```python
from build123d import *

# Parameters (mm, degrees)
ESQUISSE1_R        = 2.5
ESQUISSE1_R_2      = 1.5
BOSS_EXTRU_1_DEPTH = 3.15


with BuildPart() as part:
    # Esquisse1 → Boss.-Extru.1 (new body)
    with BuildSketch(Plane.XY):
        Polygon((3.25, 0), (5.225, -7), (16.275, -7), (18.25, 0), (21.5, 0), (21.5, 22.15), (0, 22.15), (0, 0), align=None)
        with Locations((10.75, 11.075)):
            Circle(ESQUISSE1_R, mode=Mode.SUBTRACT)
        with Locations((10.75, -1.5)):
            Circle(ESQUISSE1_R_2, mode=Mode.SUBTRACT)
    extrude(amount=BOSS_EXTRU_1_DEPTH)


solid = part.part
```
Input: part model. Units: mm. Frame: model coordinates. A direction names the side the tool comes from. Give positions to 0.01 mm unless a question says otherwise; leave off trailing zeros. Order: outer loops, then holes, each group sorted by start corner. A loop starts at its lowest first (then second) coordinate and runs counter-clockwise, first axis right, second up. Notation, with made-up numbers: (25, 44) - (69, 44) arc R24 cw to (69, 66) - close; hole circle Ø5 at (62, -32.5). An arc over 180 degrees is marked (long way). Put each result on its own line as item: value.
Item 1: Draft query along Y for faces 1 (the cylindrical face through (8.907, 12.765, 1.553)), 2 (the flat face through (11, 8, 3.15)), 3 (the flat face through (20, 0, 2)). Return one class per face: +Y half, -Y half, draft (parallel to the pull), parting line (faces both ways), or undercut.
Found:
face 1: undercut
face 2: draft
face 3: -Y half
Item 2: Section query A-A, the plane y = 10.5. Return loops of the section in (x, z).
Found:
outline: (0, 0) - (8.32, 0) - (8.32, 3.15) - (0, 3.15) - close; (13.18, 0) - (21.5, 0) - (21.5, 3.15) - (13.18, 3.15) - close
Item 3: Ray query, L1, parallel to Y at x = 10.75, z = 0.7 (3 decimals); L2, parallel to Y at x = 11.75, z = 2.75; L3, parallel to X at y = 11.75, z = 1.55. Return the intervals inside material, ascending. Write a range as from..to.
Found:
L1: y = -7..-3, 0..8.575, 13.575..22.15
L2: y = -7..-2.62, -0.38..8.78, 13.37..22.15
L3: x = 0..8.34, 13.16..21.5
Item 4: Section query B-B, the plane x = 10.75. Return loops of the section in (y, z) (3 decimals).
Found:
outline: (-7, 0) - (-3, 0) - (-3, 3.15) - (-7, 3.15) - close; (0, 0) - (8.575, 0) - (8.575, 3.15) - (0, 3.15) - close; (13.575, 0) - (22.15, 0) - (22.15, 3.15) - (13.575, 3.15) - close
Item 5: Access query for faces 4 (the flat face through (2, 0, 2)), 5 (the cylindrical face through (9.25, -1.43, 1.55)). Directions: +Z, -Z, +X, -X, +Y, -Y. A direction counts if a zero-diameter tool reaches every point of the face in a straight line with its end or side. Return the directions, or none.
Found:
face 4: +Z, -Z, -X, -Y
face 5: +Z, -Z
Item 6: Section query D-D, the plane y = -1.5. Return loops of the section in (x, z), then the cut area to 3 significant figures.
Found:
outline: (3.67, 0) - (9.25, 0) - (9.25, 3.15) - (3.67, 3.15) - close; (12.25, 0) - (17.83, 0) - (17.83, 3.15) - (12.25, 3.15) - close
area: 35.1 mm^2
Item 7: Section query C-C, the plane z = 0.4. Return loops of the section in (x, y) (3 decimals), then the cut area to 3 significant figures.
Found:
outline: (0, 0) - (3.25, 0) - (5.225, -7) - (16.275, -7) - (18.25, 0) - (21.5, 0) - (21.5, 22.15) - (0, 22.15) - close; hole circle Ø5 at (10.75, 11.075); hole circle Ø3 at (10.75, -1.5)
area: 541 mm^2
